Check sheet for the modelled part. Datum: model origin and axes. Units: mm. Coordinates: 2 decimals unless noted, no trailing zeros. Loops run counter-clockwise (first coordinate to the right, second up) from the corner with the lowest first, then second, coordinate; pieces in that order, holes last. Notation, with made-up numbers: (-28.75, 58.25) -> (25.25, 58.25) arc R26 ccw to (25.25, 86.25) -> close; hole circle Ø3 at (21, -1). An arc over 180 degrees is marked (long way). Use CSV: the item, a comma, the result in double quotes. Start each with the question number.
1. Sectioned sample at A-A, the plane z = 0. Record the cut outline in (x, y) (3 decimals).
2. Sectioned sample at C-C, the plane x = 35.5. Record the cut outline in (y, z) (3 decimals).
3. Release check for a two-part mould opening along Z. For faces 1 (the face through (25.222, -60.47, -46.367)), 2 (the face through (0, -1, -13)), 3 (the face through (25.04, -0.69, -3.1)) record: pulls with the +Z half, pulls with the -Z half, needs draft (parallel to the pull), parting line crosses it, or undercut.
4. Gauge pin test, flat ends, axial feed: pin 1 (4 mm diameter, centred on x = 24.5, y = 26, fed in from +Z); pin 2 (1 mm diameter, centred on x = 13, y = 54, fed in from +Z); pin 3 (10 mm diameter, centred on x = 24.5, z = -17.5, fed in from +Y). Record the tip position at first contact, or that the pin passes through.
5. Thickness scan on L1, parallel to Z at x = 13, y = 0 (3 decimals); L2, parallel to Z at x = 9, y = 6; L3, parallel to X at y = -23, z = -65. Record the ranges inside material, lowest first.
6. Sectioned sample at D-D, the plane x = 5.5. Record the cut outline in (y, z) (3 decimals).
```python
from build123d import *

# Parameters (mm, degrees)
F0_R     = 76.2
F0_R_2   = 3.175
F1_DEPTH = 50.8
F2_R     = 12.7
F3_R     = 12.7


with BuildPart() as f1:
    # F0 (on Right) → F1 (new body)
    with BuildSketch(Plane.YZ):
        Circle(F0_R)
        Circle(F0_R_2, mode=Mode.SUBTRACT)
    extrude(amount=F1_DEPTH)

    # F2
    f2_edges = [f1.edges().sort_by_distance(p)[0] for p in [
        (50.8, -76.2, 0),
    ]]
    fillet(f2_edges, radius=F2_R)

    # F3
    f3_edges = [f1.edges().sort_by_distance(p)[0] for p in [
        (0, -76.2, 0),
    ]]
    fillet(f3_edges, radius=F3_R)


solid = f1.part
```
Completed:
1,outline,"(0, -63.5) arc R12.7 ccw to (12.7, -76.2) -> (38.1, -76.2) arc R12.7 ccw to (50.8, -63.5) -> (50.8, -3.175) -> (0, -3.175) -> close; (0, 3.175) -> (50.8, 3.175) -> (50.8, 63.5) arc R12.7 ccw to (38.1, 76.2) -> (12.7, 76.2) arc R12.7 ccw to (0, 63.5) -> close"
2,outline,"circle Ø152.4 at (0, 0); hole circle Ø6.35 at (0, 0)"
3,face 1,"parting line crosses it"
3,face 2,"needs draft"
3,face 3,"undercut"
4,pin 1,"z = 72.32"
4,pin 2,"z = 54.26"
4,pin 3,"y = 75.17"
5,L1,"-76.2 to -3.175, 3.175 to 76.2"
5,L2,"-75.41 to 75.41"
5,L3,"1.23 to 49.57"
6,outline,"circle Ø147.924 at (0, 0); hole circle Ø6.35 at (0, 0)"
